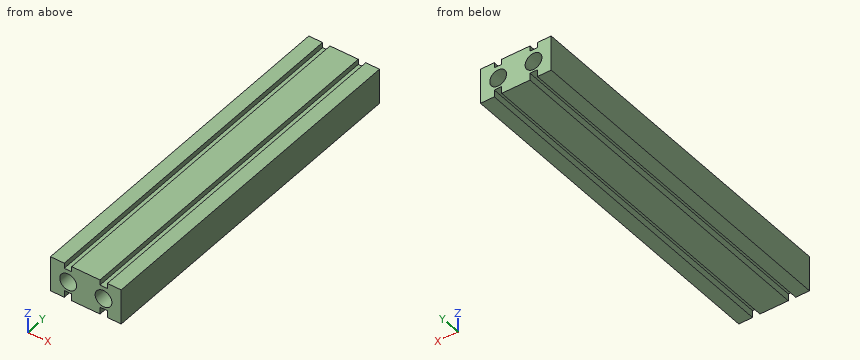
```python
from build123d import *

# Parameters (mm, degrees)
SKETCH_2_W          = 40
SKETCH_2_H          = 20
EXTRUDE_1_DEPTH     = 197
SKETCH_3_R          = 4.75
CUT_EXTRUDE_1_DEPTH = 198
SKETCH_4_W          = 4.2
SKETCH_4_H          = 197
CUT_EXTRUDE_2_DEPTH = 3
SKETCH_5_W          = 4.2
SKETCH_5_H          = 197
CUT_EXTRUDE_3_DEPTH = 4


with BuildPart() as part:
    # 草图2 → 凸台-拉伸1 (new body)
    with BuildSketch(Plane(origin=(0, 0, 0), x_dir=(1, 0, 0), z_dir=(0, 1, 0))):
        Rectangle(SKETCH_2_W, SKETCH_2_H)
    extrude(amount=EXTRUDE_1_DEPTH)

    # 草图3 → 切除-拉伸1 (cut, through all)
    with BuildSketch(Plane.XZ):
        with Locations((-10, 0)):
            Circle(SKETCH_3_R)
        with Locations((10, 0)):
            Circle(SKETCH_3_R)
    extrude(amount=-CUT_EXTRUDE_1_DEPTH, mode=Mode.SUBTRACT)

    # 草图4 → 切除-拉伸2 (cut)
    with BuildSketch(Plane.XY.offset(10)):
        with Locations((-10.1, 98.5)):
            Rectangle(SKETCH_4_W, SKETCH_4_H)
        with Locations((10.1, 98.5)):
            Rectangle(SKETCH_4_W, SKETCH_4_H)
    extrude(amount=-CUT_EXTRUDE_2_DEPTH, mode=Mode.SUBTRACT)

    # 草图5 → 切除-拉伸3 (cut)
    with BuildSketch(Plane(origin=(0, 0, -10), x_dir=(-1, 0, 0), z_dir=(0, 0, -1))):
        with Locations((-10.1, 98.5)):
            Rectangle(SKETCH_5_W, SKETCH_5_H)
        with Locations((10.1, 98.5)):
            Rectangle(SKETCH_5_W, SKETCH_5_H)
    extrude(amount=-CUT_EXTRUDE_3_DEPTH, mode=Mode.SUBTRACT)


solid = part.part
```
The model under review builds one solid part; all positions refer to its coordinate system, in mm. Round coordinates to 2 decimals unless told otherwise and drop trailing zeros. Order: outer loops, then holes, each group sorted by start corner. A loop starts at its lowest first (then second) coordinate and runs counter-clockwise, first axis right, second up. Notation, with made-up numbers: (17.5, -31) - (28.5, -31) arc R26 cw to (28.5, -13) - close; hole circle Ø10 at (-9.75, -25). An arc over 180 degrees is marked (long way). Answer in a Markdown table with one row per item.
(1) Clearance check with flat-ended pins moving along their axes: P1, Ø1.3, axis at x = -9.5, y = 106.5, coming from the -Z side; P2, Ø1.5, axis at x = -10, y = 176.5, coming from the +Z side. State where each tip first meets the part, or that it passes through.
Result set:
| item | result |
|---|---|
| P1 | stops at z = -6 |
| P2 | stops at z = 7 |
(2) Take a section at B-B on y = 145. Write out the cut boundary in (x, z).
Result set:
| item | result |
|---|---|
| outline | (-20, -10) - (-12.2, -10) - (-12.2, -6) - (-8, -6) - (-8, -10) - (8, -10) - (8, -6) - (12.2, -6) - (12.2, -10) - (20, -10) - (20, 10) - (12.2, 10) - (12.2, 7) - (8, 7) - (8, 10) - (-8, 10) - (-8, 7) - (-12.2, 7) - (-12.2, 10) - (-20, 10) - close; hole circle Ø9.5 at (-10, 0); hole circle Ø9.5 at (10, 0) |
(3) Take a section at A-A on x = 10. Write out the cut boundary in (y, z), plus the area to 4 significant figures.
Result set:
| item | result |
|---|---|
| outline | (0, -6) - (197, -6) - (197, -4.75) - (0, -4.75) - close; (0, 4.75) - (197, 4.75) - (197, 7) - (0, 7) - close |
| area | 689.5 mm2 |
(4) For line 1 (X direction, y = 90, z = 8.5); line 2 (X direction, y = 8, z = -0.25); line 3 (Z direction, x = -10, y = 150), list the stretches that pass through material, from the lowest coordinate up. Write a range as from..to.
Result set:
| item | result |
|---|---|
| line 1 | x = -20..-12.2, -8..8, 12.2..20 |
| line 2 | x = -20..-14.74, -5.26..5.26, 14.74..20 |
| line 3 | z = -6..-4.75, 4.75..7 |
(5) Take a section at C-C on z = 0. Write out the cut boundary in (x, y).
Result set:
| item | result |
|---|---|
| outline | (-20, 0) - (-14.75, 0) - (-14.75, 197) - (-20, 197) - close; (-5.25, 0) - (5.25, 0) - (5.25, 197) - (-5.25, 197) - close; (14.75, 0) - (20, 0) - (20, 197) - (14.75, 197) - close |
